from build123d import *

# Parameters (mm, degrees)
PAD_DEPTH       = 3
POCKET_DEPTH    = 2
SKETCH002_R     = 1
POCKET001_DEPTH = 5
SKETCH003_R     = 1
POCKET002_DEPTH = 5
SKETCH004_R     = 1
POCKET003_DEPTH = 5
SKETCH005_R     = 7
PAD001_DEPTH    = 15
SKETCH006_R     = 4
PAD002_DEPTH    = 7
SKETCH007_R     = 2
POCKET004_DEPTH = 5


with BuildPart() as part:
    # Sketch001 → Pad (new body)
    with BuildSketch(Plane.XY):
        with BuildLine():
            ThreePointArc((-10.37, -3.5), (-5.464747, -9.51292), (2.189111, -10.791652))
            Line((2.189111, -10.791652), (7.504111, -19.997502))
            Line((4.473022, -21.747502), (7.504111, -19.997502))
            Line((11.473022, -33.871858), (4.473022, -21.747502))
            Line((23.597378, -26.871858), (11.473022, -33.871858))
            Line((16.597378, -14.747502), (23.597378, -26.871858))
            Line((13.566289, -16.497502), (16.597378, -14.747502))
            Line((8.268243, -7.321016), (13.566289, -16.497502))
            ThreePointArc((8.268243, -7.321016), (11.058304, -0.022464), (8.298076, 7.287423))
            Line((8.298076, 7.287423), (13.613076, 16.493273))
            Line((13.613076, 16.493273), (16.644165, 14.743273))
            Line((16.644165, 14.743273), (23.644166, 26.867628))
            Line((11.519811, 33.867628), (23.644166, 26.867628))
            Line((4.519811, 21.743272), (11.519811, 33.867628))
            Line((4.519811, 21.743272), (7.5509, 19.993272))
            Line((2.233255, 10.782842), (7.5509, 19.993272))
            ThreePointArc((2.233255, 10.782842), (-5.445271, 9.524201), (-10.37, 3.5))
            Line((-21, 3.5), (-10.37, 3.5))
            Line((-21, 7), (-21, 3.5))
            Line((-35, 7), (-21, 7))
            Line((-35, -7), (-35, 7))
            Line((-21, -7), (-35, -7))
            Line((-21, -3.5), (-21, -7))
            Line((-21, -3.5), (-10.37, -3.5))
        make_face()
    extrude(amount=PAD_DEPTH)

    # Sketch (on Face26 of Pad) → Pocket (cut)
    with BuildSketch(Plane.XY.offset(3)):
        with BuildLine():
            ThreePointArc((-32.36921, -3), (-22.7, 0), (-32.36921, 3))
            Line((-36.36921, 3), (-32.36921, 3))
            Line((-36.36921, 3), (-36.36921, -3))
            Line((-36.36921, -3), (-32.36921, -3))
        make_face()
        with BuildLine():
            ThreePointArc((18.817882, -26.593527), (11.3852, -19.719745), (13.621729, -29.593527))
            Line((16.401924, -34.408965), (13.621729, -29.593527))
            Line((16.401924, -34.408965), (21.598076, -31.408965))
            Line((21.598076, -31.408965), (18.817882, -26.593527))
        make_face()
        with BuildLine():
            ThreePointArc((13.671444, 29.589525), (11.425024, 19.719543), (18.870322, 26.577421))
            Line((21.642084, 31.378253), (18.870322, 26.577421))
            Line((16.450494, 34.386142), (21.642084, 31.378253))
            Line((13.671444, 29.589525), (16.450494, 34.386142))
        make_face()
    extrude(amount=-POCKET_DEPTH, mode=Mode.SUBTRACT)

    # Sketch002 (on Face38 of Pocket) → Pocket001 (cut)
    with BuildSketch(Plane.XY.offset(1)):
        with Locations((-28, 0)):
            Circle(SKETCH002_R)
    extrude(amount=-POCKET001_DEPTH, mode=Mode.SUBTRACT)

    # Sketch003 (on Face39 of Pocket001) → Pocket002 (cut)
    with BuildSketch(Plane.XY.offset(1)):
        with Locations((14.081988, 24.30545)):
            Circle(SKETCH003_R)
    extrude(amount=-POCKET002_DEPTH, mode=Mode.SUBTRACT)

    # Sketch004 (on Face39 of Pocket002) → Pocket003 (cut)
    with BuildSketch(Plane.XY.offset(1)):
        with Locations((14.0352, -24.30968)):
            Circle(SKETCH004_R)
    extrude(amount=-POCKET003_DEPTH, mode=Mode.SUBTRACT)

    # Sketch005 (on Face5 of Pocket003) → Pad001 (join)
    with BuildSketch(Plane.XY.offset(3)):
        Circle(SKETCH005_R)
    extrude(amount=PAD001_DEPTH)

    # Sketch006 (on Face43 of Pad001) → Pad002 (join)
    with BuildSketch(Plane.XY.offset(18)):
        Circle(SKETCH006_R)
    extrude(amount=PAD002_DEPTH)

    # Sketch007 (on Face45 of Pad002) → Pocket004 (cut)
    with BuildSketch(Plane.XY.offset(25)):
        Circle(SKETCH007_R)
    extrude(amount=-POCKET004_DEPTH, mode=Mode.SUBTRACT)


solid = part.part
The listing builds one solid part. Answer for the finished solid, in the listing's coordinates (mm). A direction names the side the tool comes from. Coordinates: 2 decimals unless noted, no trailing zeros. Order: outer loops, then holes, each group sorted by start corner. A loop starts at its lowest first (then second) coordinate and runs counter-clockwise, first axis right, second up. Notation, with made-up numbers: (-20, 13.5) -> (0, 13.5) arc R7 cw to (0, 17.5) -> close; hole circle Ø1 at (5.5, 62). An arc over 180 degrees is marked (long way). Answer in a Markdown table with one row per item. Add a question column.
Item 1: Find section D-D (z = 8.5). Write down the section's boundary in (x, y).
Item 2: Find section B-B (y = 0). Write down the section's boundary in (x, z).
Item 3: Which of the six approach directions +Z, -Z, +X, -X, +Y, -Y give full straight-line access (tool end or side, diameter ignored) to faces 1 (the face through (5.967, -20.885, 1.479)), 2 (the face through (10.88, -11.845, 1.479)), 3 (the face through (6.466, -2.681, 10.395))?
Item 4: Find section C-C (x = -12). Write down the section's boundary in (y, z).
Item 5: Each of these flat-tipped pins is pushed along its axis until it touches: P1, Ø4, axis at x = -5, z = 15.5, coming from the +Y side; P2, Ø2, axis at y = 3, z = 8, coming from the +X side; P3, Ø10, axis at x = -7.5, z = 18, coming from the +Y side. Where does it stop, or does it pass through?
Item 6: Find section A-A (x = -28). Write down the section's boundary in (y, z).
Item 7: Find the intervals of material crossed by L1, parallel to Y at x = 0, z = 23.2; L2, parallel to Y at x = -28, z = 1.6; L3, parallel to X at y = 0, z = 2.3, in increasing order. Write a range as from..to.
Item 8: Determine the mould class of faces 4 (the face through (13.3, -23.63, 0.51)), 5 (the face through (7.97, 27.72, 1.48)), 6 (the face through (-2, -1, 25)) for opening direction X: +X half, -X half, draft (parallel to the pull), parting line (faces both ways), or undercut.
Result set:
| question | item | result |
|---|---|---|
| 1 | outline | circle Ø14 at (0, 0) |
| 2 | outline | (-35, 0) -> (-29, 0) -> (-29, 1) -> (-35, 1) -> close; (-27, 0) -> (11.06, 0) -> (11.06, 3) -> (7, 3) -> (7, 18) -> (4, 18) -> (4, 25) -> (2, 25) -> (2, 20) -> (-2, 20) -> (-2, 25) -> (-4, 25) -> (-4, 18) -> (-7, 18) -> (-7, 3) -> (-22.7, 3) -> (-22.7, 1) -> (-27, 1) -> close |
| 3 | face 1 | +Z, -Z, -X |
| 3 | face 2 | +Z, -Z |
| 3 | face 3 | +Z |
| 4 | outline | (-3.5, 0) -> (3.5, 0) -> (3.5, 3) -> (-3.5, 3) -> close |
| 5 | P1 | stops at y = 6.32 |
| 5 | P2 | stops at x = 6.71 |
| 5 | P3 | stops at y = 6.54 |
| 6 | outline | (-7, 0) -> (-1, 0) -> (-1, 1) -> (-5.3, 1) -> (-5.3, 3) -> (-7, 3) -> close; (1, 0) -> (7, 0) -> (7, 3) -> (5.3, 3) -> (5.3, 1) -> (1, 1) -> close |
| 7 | L1 | y = -4..-2, 2..4 |
| 7 | L2 | y = -7..-5.3, 5.3..7 |
| 7 | L3 | x = -22.7..11.06 |
| 8 | face 4 | undercut |
| 8 | face 5 | -X half |
| 8 | face 6 | draft |
